from build123d import *

# Parameters (mm, degrees)
F0_W     = 250
F0_H     = 250
F1_DEPTH = 15
F2_R     = 30
F3_DEPTH = 130


with BuildPart() as f1:
    # F0 (on Top) → F1 (new body)
    with BuildSketch(Plane.XY):
        Rectangle(F0_W, F0_H)
    extrude(amount=F1_DEPTH)

    # F2 (on face) → F3 (join)
    with BuildSketch(Plane.XZ.offset(125)):
        with BuildLine():
            Line((-17.5, 15), (-17.5, 55.709416))
            ThreePointArc((-17.5, 55.709416), (-25, 135), (-32.5, 55.709416))
            Line((-32.5, 55.709416), (-32.5, 15))
            Line((-32.5, 15), (-17.5, 15))
        make_face()
        with Locations((-25, 95)):
            Circle(F2_R, mode=Mode.SUBTRACT)
    extrude(amount=-F3_DEPTH)


solid = f1.part
Work out the finished part from the listing and answer in its coordinate system (mm). A direction names the side the tool comes from. Round coordinates to 2 decimals unless told otherwise and drop trailing zeros. Write each loop counter-clockwise with the first axis right and the second up, starting at its lowest first coordinate (ties: lowest second). Pieces come first, ordered by that corner, then holes. Notation, with made-up numbers: (-16, 56.25) -> (2, 56.25) arc R6 cw to (2, 60.25) -> close; hole circle Ø2 at (-8.75, 25.5). An arc over 180 degrees is marked (long way). Answer as CSV lines item,"result". Start each with the question number.
(1) The part is cut by section B-B, the plane z = 95. Give the vertices of the cut face in (x, y).
(2) A tool of negligible diameter and unlimited length cuts with its end or side. For faces 4 (the flat face through (-32.5, -61, 36)), 5 (the flat face through (-19, -125, 37)), from which of +Z, -Z, +X, -X, +Y, -Y can it reach the whole face along a straight path? Write none if from no direction.
(3) The mould has two halves that part along X. Classify faces 1 (the flat face through (-17.5, -61, 35)), 2 (the flat face through (-37, 5, 66)), 3 (the cylindrical face through (-28.905, -60.91, 124.745)): +X half, -X half, draft (parallel to the pull), parting line (faces both ways), or undercut.
(4) Find the intervals of material crossed by probe 1 along Z at (x, y) = (-25, -20.5); probe 2 along Z at (x, y) = (-17, -58); probe 3 along X at (y, z) = (-10, 96), in increasing order.
(5) Each of these flat-tipped pins is pushed along its axis until it touches: pin 1 (24 mm diameter, centred on x = -21, z = 102.5, fed in from +Y); pin 2 (10 mm diameter, centred on x = 54.5, y = -8.5, fed in from +Z); pin 3 (12 mm diameter, centred on y = -49, z = 38.5, fed in from +X); pin 4 (12 mm diameter, centred on y = -91.5, z = 29.5, fed in from -X). Where does it stop, or does it pass through?
(6) The part is cut by section C-C, the plane y = -39. Give the vertices of the cut face in (x, z), then the cut area to 3 significant figures.
(7) The part is cut by section A-A, the plane x = -25. Give the vertices of the cut face in (y, z).
(8) The part is cut by section D-D, the plane x = -60. Give the vertices of the cut face in (y, z).
Output values:
1,outline,"(-65, -125) -> (-55, -125) -> (-55, 5) -> (-65, 5) -> close; (5, -125) -> (15, -125) -> (15, 5) -> (5, 5) -> close"
2,face 4,"-X, +Y, -Y"
2,face 5,"+Z, -Z, +X, -X, -Y"
3,face 1,"+X half"
3,face 2,"draft"
3,face 3,"undercut"
4,probe 1,"z = 0 to 65, 125 to 135"
4,probe 2,"z = 0 to 15, 55.81 to 66.09, 123.91 to 134.19"
4,probe 3,"x = -64.99 to -54.98, 4.98 to 14.99"
5,pin 1,"passes through"
5,pin 2,"stops at z = 15"
5,pin 3,"stops at x = -17.5"
5,pin 4,"stops at x = -32.5"
6,outline,"(-125, 0) -> (125, 0) -> (125, 15) -> (-17.5, 15) -> (-17.5, 55.71) arc R40 ccw (long way) to (-32.5, 55.71) -> (-32.5, 15) -> (-125, 15) -> close; hole circle Ø60 at (-25, 95)"
6,area,"6,550 mm²"
7,outline,"(-125, 0) -> (125, 0) -> (125, 15) -> (5, 15) -> (5, 65) -> (-125, 65) -> close; (-125, 125) -> (5, 125) -> (5, 135) -> (-125, 135) -> close"
8,outline,"(-125, 0) -> (125, 0) -> (125, 15) -> (-125, 15) -> close; (-125, 75.64) -> (5, 75.64) -> (5, 114.36) -> (-125, 114.36) -> close"
